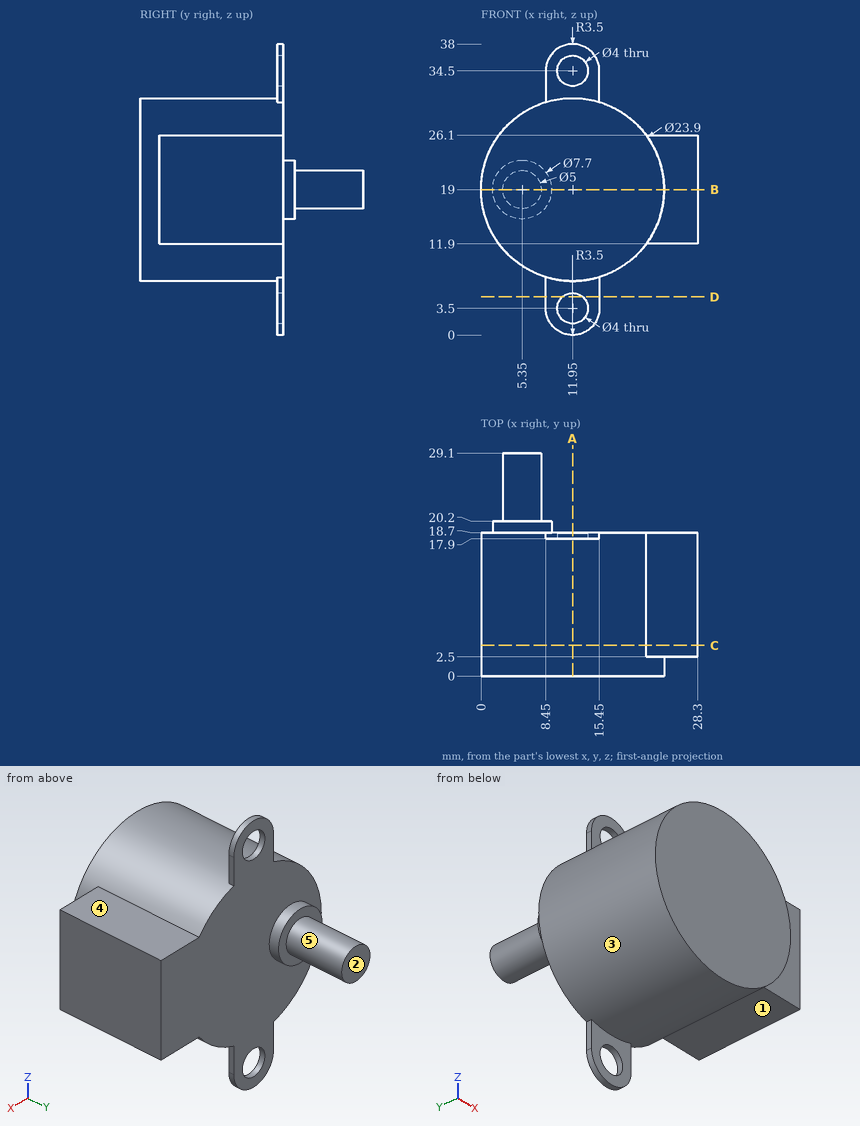
Part print with two shaded views. Sizes in mm from the minimum x, y, z corner. A direction names the side the tool comes from. Round coordinates to 2 decimals unless told otherwise and drop trailing zeros. Order: outer loops, then holes, each group sorted by start corner. A loop starts at its lowest first (then second) coordinate and runs counter-clockwise, first axis right, second up.
(1) Band-saw the part on D-D (z = 5). List the corners of the cut face in (x, y), then the cut area to 3 significant figures.
(2) Band-saw the part on B-B (z = 19). List the corners of the cut face in (x, y).
(3) Band-saw the part on A-A (x = 11.95). List the corners of the cut face in (y, z), then the cut area to 3 significant figures.
(4) Band-saw the part on C-C (y = 4). List the corners of the cut face in (x, z).
(5) Pin check, flat tips, straight feed: pin 1 (6 mm diameter, centred on x = 8.5, z = 4, fed in from -Y); pin 2 (4 mm diameter, centred on x = 5.5, y = 20.5, fed in from +Z); pin 3 (7.5 mm diameter, centred on x = 12.5, z = 5.5, fed in from -Y); pin 4 (3.5 mm diameter, centred on x = 26.5, y = 11.5, fed in from -Z). Stop position of each tip, or through.
(6) Drill centre lines: line 1 (Y direction, x = 27, z = 19.5); line 2 (X direction, y = 18.1, z = 3.5); line 3 (Y direction, x = 8.5, z = 30). Where is each one in solid material? Low to high.
(7) 3-axis set-ups, long thin cutter, end or side, ignore diameter. For the marked faces 1, 2, 3, 4 and 5: which of +Z, -Z, +X, -X, +Y, -Y reach the whole face in a straight line?
Verdict:
1. outline: (8.45, 17.9) - (10.63, 17.9) - (10.63, 18.7) - (8.45, 18.7) - close; (13.27, 17.9) - (15.45, 17.9) - (15.45, 18.7) - (13.27, 18.7) - close
1. area: 3.48 mm2
2. outline: (0, 0) - (23.9, 0) - (23.9, 2.5) - (28.3, 2.5) - (28.3, 18.7) - (9.2, 18.7) - (9.2, 20.2) - (7.85, 20.2) - (7.85, 29.1) - (2.85, 29.1) - (2.85, 20.2) - (1.5, 20.2) - (1.5, 18.7) - (0, 18.7) - close
3. outline: (0, 7.05) - (17.9, 7.05) - (17.9, 5.5) - (18.7, 5.5) - (18.7, 32.5) - (17.9, 32.5) - (17.9, 30.95) - (0, 30.95) - close; (17.9, 0) - (18.7, 0) - (18.7, 1.5) - (17.9, 1.5) - close; (17.9, 36.5) - (18.7, 36.5) - (18.7, 38) - (17.9, 38) - close
3. area: 452 mm2
4. outline: (21.56, 11.9) - (28.3, 11.9) - (28.3, 26.1) - (21.56, 26.1) arc R11.95 ccw (long way) to start
5. pin 1: stops at y = 17.9
5. pin 2: stops at z = 29.57
5. pin 3: stops at y = 0
5. pin 4: stops at z = 11.9
6. line 1: y = 2.5 to 18.7
6. line 2: x = 8.45 to 9.95, 13.95 to 15.45
6. line 3: y = 0 to 18.7
7. face 1: -Z, +X, +Y, -Y
7. face 2: +Z, -Z, +X, -X, +Y
7. face 3: -Y
7. face 4: +Z, +X, +Y, -Y
7. face 5: +Y
